```python
from build123d import *

# Parameters (mm, degrees)
SKETCH1_R           = 20.9
BOSS_EXTRUDE1_DEPTH = 30.75
CHAMFER1_SIZE       = 5
CHAMFER1_SIZE2      = 6
CHAMFER2_SIZE       = 2
CHAMFER2_SIZE2      = 5.494954839
SKETCH2_R           = 2
BOSS_EXTRUDE2_DEPTH = 5.5
SKETCH3_R           = 4
BOSS_EXTRUDE3_DEPTH = 2.55


with BuildPart() as part:
    # Sketch1 → Boss-Extrude1 (new body)
    with BuildSketch(Plane(origin=(0, 0, 0), x_dir=(1, 0, 0), z_dir=(0, 1, 0))):
        with Locations(Location((-5.649057894, -5.328088696, 0), (0, 0, 270))):
            Circle(SKETCH1_R)
    extrude(amount=BOSS_EXTRUDE1_DEPTH)

    # Chamfer1
    chamfer1_edges = [part.edges().sort_by_distance(p)[0] for p in [
        (-5.649057894, 30.75, -15.571911304),
    ]]
    chamfer1_side = [part.faces().sort_by_distance(p)[0] for p in [
        (-5.649057894, 15.375, -15.571911304),
    ]]
    chamfer(chamfer1_edges, length=CHAMFER1_SIZE, length2=CHAMFER1_SIZE2, reference=chamfer1_side[0])

    # Chamfer2
    chamfer2_edges = [part.edges().sort_by_distance(p)[0] for p in [
        (-5.649057894, 0, -15.571911304),
    ]]
    chamfer2_side = [part.faces().sort_by_distance(p)[0] for p in [
        (-5.649057894, 0, 5.328088696),
    ]]
    chamfer(chamfer2_edges, length=CHAMFER2_SIZE, length2=CHAMFER2_SIZE2, reference=chamfer2_side[0])

    # Sketch2 → Boss-Extrude2 (add)
    with BuildSketch(Plane(origin=(0, 30.75, 0), x_dir=(1, 0, 0), z_dir=(0, 1, 0))):
        with Locations(Location((-5.649057894, -5.328088696, 0), (0, 0, 270))):
            Circle(SKETCH2_R)
    extrude(amount=BOSS_EXTRUDE2_DEPTH)

    # Sketch3 → Boss-Extrude3 (add)
    with BuildSketch(Plane.XZ):
        with Locations(Location((-5.649057894, 5.328088696, 0), (0, 0, 90))):
            Circle(SKETCH3_R)
    extrude(amount=BOSS_EXTRUDE3_DEPTH)


solid = part.part
```
Can you work these out from the model? Positions are in its coordinate system, mm. A direction names the side the tool comes from. Coordinates: 2 decimals unless noted, no trailing zeros. Loops run counter-clockwise (first coordinate to the right, second up) from the corner with the lowest first, then second, coordinate; pieces in that order, holes last. Notation, with made-up numbers: M 23,68 L 53,68 A28 cw 53,100 Z; hole C 76,71 d7. An arc over 180 degrees is marked long. Put each result on its own line as item: value. Start each with the question number.
(1) Which directions (+Z, -Z, +X, -X, +Y, -Y) give clear straight access to the entire face, cutting with the end or side of a thin tool? Please do faces 1 (the face through (-2.1, -1.26, 7.17)), 2 (the face through (-7.423, 33.462, 6.251)), 3 (the face through (-6, 36.25, 5)).
(2) I need wall thicknesses on probe 1 along Y at (x, z) = (0.5, -0.5); probe 2 along Z at (x, y) = (-23, 24); probe 3 along X at (y, z) = (14, 22). Which ranges of each line are inside material? Lowest first, please.
(3) Imagine slicing it at A-A on y = 28. List the corners of the cut face in (x, z) for me, and give its area (3 significant figures).
(4) Imagine slicing it at B-B on y = 3. List the corners of the cut face in (x, z) for me, and give its area (3 significant figures).
(5) Will these pins go through, and if not, where does the flat tip stop? pin 1 Ø1.5 at (x, z) = (-12, 8.5) entering from -Y; pin 2 Ø6 at (y, z) = (20, 19) entering from -X; pin 3 Ø3 at (x, y) = (-15.5, 18) entering from -Z.
Worked answers:
1. face 1: -Y
1. face 2: +Y
1. face 3: +Z, -Z, +X, -X, +Y
2. probe 1: y = 0 to 30.75
2. probe 2: z = -6.32 to 16.98
2. probe 3: x = -18.25 to 6.95
3. outline: C -5.65,5.33 d36.4
3. area: 1,040 mm2
4. outline: C -5.65,5.33 d39.98
4. area: 1,260 mm2
5. pin 1: stops at y = 0
5. pin 2: stops at x = -23.62
5. pin 3: stops at z = -13.83
